from build123d import *

# Parameters (mm, degrees)
BOSS_EXTRU_1_DEPTH      = 10
BOSS_EXTRU_2_DEPTH      = 48
BOSS_EXTRU_3_DEPTH      = 2
CHANFREIN1_SIZE         = 6
ENL_V_MAT_EXTRU_1_REACH = 148.244
ESQUISSE5_R             = 1.75
ESQUISSE6_R             = 3.5
ENL_V_MAT_EXTRU_2_DEPTH = 4
CHANFREIN2_SIZE         = 7.5
ESQUISSE7_R             = 1.25
ENL_V_MAT_EXTRU_3_DEPTH = 10
BOSS_EXTRU_4_DEPTH      = 10
ESQUISSE9_R             = 2.75
ENL_V_MAT_EXTRU_4_DEPTH = 2


with BuildPart() as part:
    # Esquisse1 → Boss.-Extru.1 (new body)
    with BuildSketch(Plane.XY):
        with BuildLine():
            Line((-40.181760398, -97.007350914), (-47.835429046, -115.484941564))
            ThreePointArc((-47.835429046, -115.484941564), (-24.386290252, -122.59816005), (0, -125))
            Line((0, -125), (0, -105))
            ThreePointArc((0, -105), (-20.484483812, -102.982454442), (-40.181760398, -97.007350914))
        make_face()
    extrude(amount=BOSS_EXTRU_1_DEPTH)

    # Esquisse2 → Boss.-Extru.2 (add)
    with BuildSketch(Plane.XY.offset(10)):
        with BuildLine():
            Line((-32.925344295, -102.858746361), (-38.108037379, -119.049474955))
            ThreePointArc((-38.108037379, -119.049474955), (-24.386290252, -122.59816005), (-10.351025939, -124.570687812))
            Line((-10.351025939, -124.570687812), (-8.943286411, -107.62907427))
            ThreePointArc((-8.943286411, -107.62907427), (-21.069754778, -105.924810284), (-32.925344295, -102.858746361))
        make_face()
    extrude(amount=BOSS_EXTRU_2_DEPTH)

    # Esquisse4 → Boss.-Extru.3 (add)
    with BuildSketch(Plane.XY.offset(58)):
        with BuildLine():
            Line((-39.413172773, -123.12671677), (-10.705530953, -128.837021766))
            Line((-10.705530953, -128.837021766), (-8.943286411, -107.62907427))
            ThreePointArc((-8.943286411, -107.62907427), (-21.069754778, -105.924810284), (-32.925344295, -102.858746361))
            Line((-32.925344295, -102.858746361), (-39.413172773, -123.12671677))
        make_face()
    extrude(amount=BOSS_EXTRU_3_DEPTH)

    # Chanfrein1
    # the kernel refuses this chamfer: 6 mm, written as the material it adds along each edge
    with BuildSketch(Plane(origin=(0, 0, 58), x_dir=(-0.3048642990280114, -0.9523957996432781, 0), z_dir=(-0.9523957996432781, 0.3048642990280114, 0))) as chanfrein1_piece_1_section:
        Polygon((125 + CHANFREIN1_SIZE, 0), (125, -CHANFREIN1_SIZE), (125, 0), align=None)
    chanfrein1_piece_1 = revolve(axis=Axis((0, 0, 58), (0, 0, 1)), revolution_arc=13, mode=Mode.PRIVATE)
    chanfrein1_piece_1 = split(chanfrein1_piece_1, bisect_by=Plane(origin=(-25.059351863, -125.981869268, 58), z_dir=(0.19509032201612828, 0.9807852804032304, 0)), keep=Keep.TOP, mode=Mode.PRIVATE)
    add(chanfrein1_piece_1)

    # Esquisse5 → Enlèv. mat.-Extru.1 (cut, up to next)
    with BuildSketch(Plane.XY.offset(10), mode=Mode.PRIVATE) as enl_v_mat_extru_1_sk1:
        with Locations((-4.765565521, -114.901215769)):
            Circle(ESQUISSE5_R)
    enl_v_mat_extru_1_tool1 = extrude(enl_v_mat_extru_1_sk1.sketch, amount=-ENL_V_MAT_EXTRU_1_REACH, mode=Mode.PRIVATE) & part.part
    # Esquisse5 → Enlèv. mat.-Extru.1 (cut, up to next)
    with BuildSketch(Plane.XY.offset(10), mode=Mode.PRIVATE) as enl_v_mat_extru_1_sk2:
        with Locations((-39.567983188, -107.978584481)):
            Circle(ESQUISSE5_R)
    enl_v_mat_extru_1_tool2 = extrude(enl_v_mat_extru_1_sk2.sketch, amount=-ENL_V_MAT_EXTRU_1_REACH, mode=Mode.PRIVATE) & part.part
    add(enl_v_mat_extru_1_tool1.solids().sort_by_distance((-4.765566, -114.901216, 10))[0], mode=Mode.SUBTRACT)
    add(enl_v_mat_extru_1_tool2.solids().sort_by_distance((-39.567983, -107.978584, 10))[0], mode=Mode.SUBTRACT)

    # Esquisse6 → Enlèv. mat.-Extru.2 (cut)
    with BuildSketch(Plane.XY.offset(10)):
        with Locations((-39.567983188, -107.978584481)):
            Circle(ESQUISSE6_R)
        with Locations((-4.765565521, -114.901215769)):
            Circle(ESQUISSE6_R)
    extrude(amount=-ENL_V_MAT_EXTRU_2_DEPTH, mode=Mode.SUBTRACT)

    # Chanfrein2
    # the kernel refuses this chamfer: 7.5 mm, written as the material it takes off along each edge
    with BuildSketch(Plane(origin=(-8.943286411, -107.62907427, 10), x_dir=(-0.08280820751335238, -0.996565502497666, 0), z_dir=(0, 0, 1)), Plane(origin=(-32.925344295, -102.858746361, 80.019854797), x_dir=(-0.3048642990290983, -0.9523957996429303, 0), z_dir=(0, 0, -1))) as chanfrein2_piece_1:
        with BuildLine():
            Line((CHANFREIN2_SIZE, 0), (-0.280634385, -7.780634385))
            ThreePointArc((-0.280634385, -7.780634385), (-0.074202159, -4.002769088), (0, 0))
            Line((0, 0), (CHANFREIN2_SIZE, 0))
        make_face()
    extrude(amount=70.019854797, mode=Mode.SUBTRACT)

    # Esquisse7 → Enlèv. mat.-Extru.3 (cut)
    with BuildSketch(Plane.XY.offset(60)):
        with Locations((-30.083912118, -112.798307752)):
            Circle(ESQUISSE7_R)
        with Locations((-15.372132912, -115.724662582)):
            Circle(ESQUISSE7_R)
    extrude(amount=-ENL_V_MAT_EXTRU_3_DEPTH, mode=Mode.SUBTRACT)

    # Esquisse8 → Boss.-Extru.4 (add)
    with BuildSketch(Plane(origin=(0, 0, 0), x_dir=(-1, 0, 0), z_dir=(0, 0, -1))):
        with BuildLine():
            Line((22.625550905, -139.375480075), (32.433403709, -137.424576855))
            Line((32.433403709, -137.424576855), (38.108037379, -119.049474955))
            ThreePointArc((38.108037379, -119.049474955), (24.386290252, -122.59816005), (10.351025939, -124.570687812))
            Line((10.351025939, -124.570687812), (22.625550905, -139.375480075))
        make_face()
    extrude(amount=-BOSS_EXTRU_4_DEPTH)

    # Esquisse9 → Enlèv. mat.-Extru.4 (cut)
    with BuildSketch(Plane(origin=(-27.529477307, -138.400028465, 0), x_dir=(0.9807852804032304, -0.19509032201612822, 0), z_dir=(-0.19509032201612822, -0.9807852804032304, 0))):
        with Locations((0, 5)):
            Circle(ESQUISSE9_R)
    extrude(amount=-ENL_V_MAT_EXTRU_4_DEPTH, mode=Mode.SUBTRACT)


solid = part.part
Verification items for the finished model (mm, model axes). A direction names the side the tool comes from. Give positions to 0.01 mm unless a question says otherwise; leave off trailing zeros. Order: outer loops, then holes, each group sorted by start corner. A loop starts at its lowest first (then second) coordinate and runs counter-clockwise, first axis right, second up. Notation, with made-up numbers: M -24.75,-27.75 L -3.75,-27.75 A25 ccw -3.75,6.25 Z; hole C -2.5,42.5 d9. An arc over 180 degrees is marked long. Use one line per item in the form item = value. Start each with the question number.
Q1. Section check A-A (z = 53). Enter the section's corners in (x, y).
Q2. Access from +Z, -Z, +X, -X, +Y, -Y to the whole of each face (thin tool, end or side, straight path). Record for faces 4 (the flat face through (-39, -106, 6)), 5 (the conical face through (-24.9, -124.16, 53.63)), 6 (the flat face through (-30.39, -107.52, 35.35)).
Q3. Scan lines: line 1 along Z through (x, y) = (-37, -100); line 2 along Z through (x, y) = (-27, -123); line 3 along Y through (x, z) = (-23, 35.5). Record each from-to range of solid material in increasing order. Write a range as [from, to].
Q4. Section check C-C (z = 8.5). Enter the section's corners in (x, y).
Q5. Section check B-B (z = 34.5). Enter the section's corners in (x, y), then the cut area to 3 significant figures.
Q6. Mould release check, pull along Z, two halves, no side actions. Record for faces 1 (the flat face through (-19, -106, 10)), 2 (the flat face through (-27, -129, 10)), 3 (the cylindrical face through (-21.008, -105.937, 34.65)): +Z half, -Z half, draft (parallel to the pull), parting line (faces both ways), or undercut.
Q7. Go/stop test with flat-tipped pins: pin 1 Ø3 at (x, z) = (-40, 26) entering from +Y; pin 2 Ø3.5 at (x, y) = (-38.5, -109) entering from +Z; pin 3 Ø5 at (x, y) = (-6.5, -116.5) entering from +Z; pin 4 Ø1.5 at (x, z) = (-13.5, 42) entering from +Y. Record where each tip stops, or that it passes through.
Evaluation:
q1.outline = M -38.41,-120 A126 ccw -10.43,-125.57 L -9.56,-115.1 L -16.67,-106.71 A108 cw -25.43,-104.96 L -35.21,-110 Z; hole C -30.08,-112.8 d2.5; hole C -15.37,-115.72 d2.5
q2.face_4 = +Z
q2.face_5 = -X, -Y
q2.face_6 = +Z, -X, +Y
q3.line_1 = [0, 10]
q3.line_2 = [0, 10], [52.93, 60]
q3.line_3 = [-122.87, -105.52]
q4.outline = M -47.84,-115.48 A125 ccw -38.11,-119.05 L -32.43,-137.42 L -22.63,-139.38 L -10.35,-124.57 A125 ccw 0,-125 L 0,-105 A105 cw -40.18,-97.01 Z; hole C -39.57,-107.98 d7; hole C -4.77,-114.9 d7
q5.outline = M -38.11,-119.05 A125 ccw -10.35,-124.57 L -9.56,-115.1 L -16.67,-106.71 A108 cw -25.43,-104.96 L -35.21,-110 Z
q5.area = 392 mm2
q6.face_1 = +Z half
q6.face_2 = undercut
q6.face_3 = draft
q7.pin_1 = through
q7.pin_2 = 6
q7.pin_3 = 10
q7.pin_4 = -109.57
